The listing builds one solid part. Answer for the finished solid, in the listing's coordinates (mm). A direction names the side the tool comes from. Give positions to 0.01 mm unless a question says otherwise; leave off trailing zeros. Order: outer loops, then holes, each group sorted by start corner. A loop starts at its lowest first (then second) coordinate and runs counter-clockwise, first axis right, second up. Notation, with made-up numbers: (-12, 88) - (11, 88) arc R12 cw to (11, 104) - close; hole circle Ø2 at (-23.75, 9). An arc over 180 degrees is marked (long way). Write each question's results on one line, items separated by ' | '. Start each with the question number.
1. Section D-D (x = -1.5) is taken. Give the vertices of the cut face in (y, z).
2. Which of the six approach directions +Z, -Z, +X, -X, +Y, -Y give full straight-line access (tool end or side, diameter ignored) to faces 1 (the face through (-19.325, 10.534, 39.44)), 2 (the face through (28.941, -19, 39)), 3 (the face through (4, -11.26, 39))?
3. Determine the mould class of faces 4 (the face through (4, 6, 0)), 5 (the face through (14.917, 0, 39)), 6 (the face through (-19.393, -10.534, 39.44)), 7 (the face through (-7.036, 0, 39)) for opening direction X: released by +X, released by -X, zero draft, split by the parting line, or undercut.
4. Section C-C (x = 20) is taken. Give the vertices of the cut face in (y, z), and give its area (3 significant figures).
5. Section A-A (x = 7) is taken. Give the vertices of the cut face in (y, z).
6. Flat-ended cylindrical pins translate along their axes: pin 1 (5.5 mm diameter, centred on x = 0.5, z = 22, fed in from -Y); pin 2 (2 mm diameter, centred on x = 4, z = 11.5, fed in from +Y); pin 3 (8.5 mm diameter, centred on y = 2, z = 38, fed in from +X). Find the tip coordinate at first contact, or state that the pin passes through.
7. Find the intervals of material crossed by L1, parallel to Y at x = 5, z = 37; L2, parallel to X at y = 2.5, z = 62; L3, parallel to X at y = 23.5, z = 35, in increasing order.
8. Section B-B (y = -17) is taken. Give the vertices of the cut face in (x, z), and give its area (3 significant figures).
from build123d import *

# Parameters (mm, degrees)
SKETCH1_W           = 50
SKETCH1_H           = 50
BOSS_EXTRUDE1_DEPTH = 80
SKETCH2_W           = 18
SKETCH2_H           = 18
CUT_EXTRUDE2_DEPTH  = 287
SKETCH3_OUTSIDE_W   = 73.354
SKETCH3_OUTSIDE_H   = 73.354
CUT_EXTRUDE5_DEPTH  = 287
SKETCH4_W           = 18
SKETCH4_H           = 18
BOSS_EXTRUDE2_DEPTH = 80
SKETCH5_W           = 8
SKETCH5_H           = 7.553245746
CUT_EXTRUDE6_DEPTH  = 250


with BuildPart() as part:
    # Sketch1 → Boss-Extrude1 (new body)
    with BuildSketch(Plane.XY):
        with Locations((3.9408867, 0)):
            Rectangle(SKETCH1_W, SKETCH1_H)
    extrude(amount=BOSS_EXTRUDE1_DEPTH)

    # Sketch2 → Cut-Extrude2 (cut)
    with BuildSketch(Plane(origin=(0, 0, 0), x_dir=(-1, 0, 0), z_dir=(0, 0, -1))):
        with Locations((-3.9408867, 0)):
            Rectangle(SKETCH2_W, SKETCH2_H)
    extrude(amount=-CUT_EXTRUDE2_DEPTH, mode=Mode.SUBTRACT)

    # Sketch3 outside → Cut-Extrude5 (cut)
    with BuildSketch(Plane(origin=(0, 0, 0), x_dir=(-1, 0, 0), z_dir=(0, 0, -1))):
        with Locations((-3.941, 0)):
            Rectangle(SKETCH3_OUTSIDE_W, SKETCH3_OUTSIDE_H)
        with BuildLine():
            Line((-22.316271067, 21.584230763), (-17.116271067, 21.584230763))
            ThreePointArc((-17.116271067, 21.584230763), (-15.082817857, 22.96654679), (-16.465133883, 25))
            Line((-16.465133883, 25), (-28.9408867, 25))
            Line((-28.9408867, 25), (-28.9408867, 12.5))
            ThreePointArc((-28.9408867, 12.5), (-27.489165976, 10.551720724), (-25.5408867, 12.003441448))
            Line((-25.5408867, 12.003441448), (-25.5408867, 20.003441448))
            Line((-25.5408867, 20.003441448), (-18.539469589, 11.659477453))
            Line((-18.539469589, 11.659477453), (-14.917465737, 7.34294135))
            Line((-14.917465737, 7.34294135), (-14.917465737, -7.34294135))
            Line((-14.917465737, -7.34294135), (-18.539469589, -11.659477453))
            Line((-18.539469589, -11.659477453), (-25.5408867, -20.003441448))
            Line((-25.5408867, -20.003441448), (-25.5408867, -12.003441448))
            ThreePointArc((-25.5408867, -12.003441448), (-27.489165976, -10.551720724), (-28.9408867, -12.5))
            Line((-28.9408867, -12.5), (-28.9408867, -25))
            Line((-28.9408867, -25), (-16.465133883, -25))
            ThreePointArc((-16.465133883, -25), (-15.082817857, -22.96654679), (-17.116271067, -21.584230763))
            Line((-17.116271067, -21.584230763), (-22.316271067, -21.584230763))
            Line((-22.316271067, -21.584230763), (-17.28167328, -15.584230763))
            Line((-17.28167328, -15.584230763), (-13.653142176, -11.259915785))
            Line((-13.653142176, -11.259915785), (5.089795616, -11.259915785))
            Line((5.089795616, -11.259915785), (8.71832672, -15.584230763))
            Line((8.71832672, -15.584230763), (13.752924507, -21.584230763))
            Line((13.752924507, -21.584230763), (8.5591133, -21.584230763))
            ThreePointArc((8.5591133, -21.584230763), (6.851228682, -23.292115382), (8.5591133, -25))
            Line((8.5591133, -25), (21.0591133, -25))
            Line((21.0591133, -25), (21.0591133, -12.5))
            ThreePointArc((21.0591133, -12.5), (19.607392577, -10.551720724), (17.6591133, -12.003441448))
            Line((17.6591133, -12.003441448), (17.6591133, -20.003441448))
            Line((17.6591133, -20.003441448), (10.65769619, -11.659477453))
            Line((10.65769619, -11.659477453), (7.035692338, -7.34294135))
            Line((7.035692338, -7.34294135), (7.035692338, 7.34294135))
            Line((7.035692338, 7.34294135), (10.65769619, 11.659477453))
            Line((10.65769619, 11.659477453), (17.6591133, 20.003441448))
            Line((17.6591133, 20.003441448), (17.6591133, 12.003441448))
            ThreePointArc((17.6591133, 12.003441448), (19.607392577, 10.551720724), (21.0591133, 12.5))
            Line((21.0591133, 12.5), (21.0591133, 25))
            Line((21.0591133, 25), (8.5591133, 25))
            ThreePointArc((8.5591133, 25), (6.851228682, 23.292115382), (8.5591133, 21.584230763))
            Line((8.5591133, 21.584230763), (13.752924507, 21.584230763))
            Line((13.752924507, 21.584230763), (8.71832672, 15.584230763))
            Line((8.71832672, 15.584230763), (4.653605138, 10.740084215))
            Line((4.653605138, 10.740084215), (-13.216951698, 10.740084215))
            Line((-13.216951698, 10.740084215), (-17.28167328, 15.584230763))
            Line((-17.28167328, 15.584230763), (-22.316271067, 21.584230763))
        make_face(mode=Mode.SUBTRACT)
    extrude(amount=-CUT_EXTRUDE5_DEPTH, mode=Mode.SUBTRACT)

    # Sketch4 → Boss-Extrude2 (add)
    with BuildSketch(Plane(origin=(0, 0, 0), x_dir=(-1, 0, 0), z_dir=(0, 0, -1))):
        with Locations((-3.9408867, 0)):
            Rectangle(SKETCH4_W, SKETCH4_H)
    extrude(amount=-BOSS_EXTRUDE2_DEPTH)

    # Sketch5 → Cut-Extrude6 (cut)
    with BuildSketch(Plane(origin=(0, 0, 0), x_dir=(-1, 0, 0), z_dir=(0, 0, -1))):
        with Locations((-3.917465737, 0)):
            Rectangle(SKETCH5_W, SKETCH5_H)
    extrude(amount=-CUT_EXTRUDE6_DEPTH, mode=Mode.SUBTRACT)


solid = part.part
Reported:
1) outline: (-11.26, 0) - (10.74, 0) - (10.74, 80) - (-11.26, 80) - close
2) face 1: +Z, -Z | face 2: +Z, -Z, +X, +Y, -Y | face 3: +Z, -Z, -Y
3) face 4: zero draft | face 5: released by +X | face 6: undercut | face 7: released by -X
4) outline: (-25, 0) - (-21.58, 0) - (-21.58, 80) - (-25, 80) - close; (-18.82, 0) - (-13.4, 0) - (-13.4, 80) - (-18.82, 80) - close; (13.4, 0) - (18.82, 0) - (18.82, 80) - (13.4, 80) - close; (21.58, 0) - (25, 0) - (25, 80) - (21.58, 80) - close | area: 1,410 mm²
5) outline: (-11.26, 0) - (-3.78, 0) - (-3.78, 80) - (-11.26, 80) - close; (3.78, 0) - (10.74, 0) - (10.74, 80) - (3.78, 80) - close
6) pin 1: y = -11.26 | pin 2: y = 10.74 | pin 3: x = 14.92
7) L1: -11.26 to -3.78, 3.78 to 10.74 | L2: -7.04 to -0.08, 7.92 to 14.92 | L3: -21.06 to -6.86, 15.06 to 28.94
8) outline: (-21.06, 0) - (-17.66, 0) - (-17.66, 80) - (-21.06, 80) - close; (-15.14, 0) - (-9.91, 0) - (-9.91, 80) - (-15.14, 80) - close; (18.47, 0) - (23.02, 0) - (23.02, 80) - (18.47, 80) - close; (25.54, 0) - (28.94, 0) - (28.94, 80) - (25.54, 80) - close | area: 1,330 mm²
